Read the model definition and answer for the solid it produces. Units are mm, in the model's axes. Face numbers are marked on the shaded views. A direction names the side the tool comes from. Give positions to 0.01 mm unless a question says otherwise; leave off trailing zeros. Order: outer loops, then holes, each group sorted by start corner. A loop starts at its lowest first (then second) coordinate and runs counter-clockwise, first axis right, second up. Notation, with made-up numbers: (72, 81.25) -> (120, 81.25) arc R17 cw to (120, 95.25) -> close; hole circle Ø11 at (-38, 47.5). An arc over 180 degrees is marked (long way). Answer as CSV lines item,"result". Start each with the question number.
1) Find section C-C (y = 10). Determine the outline of the cut face in (x, z).
2) Straight lines are drawn through the part: L1, parallel to Z at x = 59.5, y = 3; L2, parallel to Y at x = 30, z = -3.7; L3, parallel to X at y = -18, z = -42.5. For each, find the intervals that lie inside material, in ascending order. Write a range as from..to.
3) The mould has two halves that part along X. Classify the marked faces 4, 5 and 6: +X half, -X half, draft (parallel to the pull), parting line (faces both ways), or undercut.
4) Find section D-D (x = 75). State how many separate pieces and enclosed holes the cut face has, and give its area (3 significant figures).
5) Find section B-B (z = -98.5). Determine the outline of the cut face in (x, y), and give its area (3 significant figures).
6) Find section A-A (y = 0). Determine the outline of the cut face in (x, z), and give its area (3 significant figures).
7) For the marked faces 1, 2 and 3, determine the directions among +Z, -Z, +X, -X, +Y, -Y from which every point of the face is accessible in a straight line to the end or side of a thin tool.
8) Flat-ended cylindrical pins translate along their axes: pin 1 Ø2.5 at (x, y) = (3.5, -7) entering from -Z; pin 2 Ø13.5 at (y, z) = (-7, -70.5) entering from +X; pin 3 Ø4 at (y, z) = (8.5, -46) entering from -X. Find the tip coordinate at first contact, or state that the pin passes through.
```python
from build123d import *

# Parameters (mm, degrees)
SKETCH1_W           = 65
SKETCH1_H           = 162
BOSS_EXTRUDE1_DEPTH = 42.5
CUT_EXTRUDE1_DEPTH  = 206.949629764
CUT_EXTRUDE2_REACH  = 207.95
SKETCH4_R           = 4.25
SKETCH5_W           = 2
SKETCH5_H           = 65
CUT_EXTRUDE3_DEPTH  = 206.949629919
CHAMFER1_SIZE       = 20


with BuildPart() as part:
    # Sketch1 → Boss-Extrude1 (new, symmetric)
    with BuildSketch(Plane(origin=(0, 0, 0), x_dir=(1, 0, 0), z_dir=(0, 1, 0))):
        Polygon((100, 5), (100, 167), (105, 172), (0, 172), (5, 167), (5, 5), (0, 5), (0, 0), (105, 0), (105, 5), align=None)
        with Locations((52.5, 86)):
            Rectangle(SKETCH1_W, SKETCH1_H, mode=Mode.SUBTRACT)
    extrude(amount=BOSS_EXTRUDE1_DEPTH, both=True)

    # Sketch2 → Cut-Extrude1 (cut, through all)
    with BuildSketch(Plane(origin=(0, 0, 0), x_dir=(0, 0, -1), z_dir=(1, 0, 0))):
        Polygon((0, 22.5), (147, 22.5), (167, 42.5), (0, 42.5), align=None)
    cut_extrude1 = extrude(amount=CUT_EXTRUDE1_DEPTH, mode=Mode.SUBTRACT)

    # Mirror1: Cut-Extrude1 across plane
    add(cut_extrude1.mirror(Plane.ZX), mode=Mode.SUBTRACT)

    # Sketch3 → section 0 of cut_loft1
    with BuildSketch(Plane(origin=(0, 0, -170), x_dir=(-1, 0, 0), z_dir=(0, 0, -1)), mode=Mode.PRIVATE) as cut_loft1_s0:
        with BuildLine():
            Line((-102.5, 40), (0, 40))
            Line((0, 40), (0, -40))
            Line((0, -40), (-102.5, -40))
            Line((-102.5, -40), (-102.5, 40))
        make_face()
    # loft up to a face of the part (cut_loft1)
    loft([cut_loft1_s0.sketch, part.faces().sort_by_distance((52.5, 0, -172))[0]], mode=Mode.SUBTRACT)

    # Sketch4 → Cut-Extrude2 (cut, up to next)
    with BuildSketch(Plane.XY, mode=Mode.PRIVATE) as cut_extrude2_sk1:
        with Locations((30, 0)):
            Circle(SKETCH4_R)
    cut_extrude2_tool1 = extrude(cut_extrude2_sk1.sketch, amount=-CUT_EXTRUDE2_REACH, mode=Mode.PRIVATE) & part.part
    # Sketch4 → Cut-Extrude2 (cut, up to next)
    with BuildSketch(Plane.XY, mode=Mode.PRIVATE) as cut_extrude2_sk2:
        with Locations((75, 0)):
            Circle(SKETCH4_R)
    cut_extrude2_tool2 = extrude(cut_extrude2_sk2.sketch, amount=-CUT_EXTRUDE2_REACH, mode=Mode.PRIVATE) & part.part
    add(cut_extrude2_tool1.solids().sort_by_distance((30, 0, 0))[0], mode=Mode.SUBTRACT)
    add(cut_extrude2_tool2.solids().sort_by_distance((75, 0, 0))[0], mode=Mode.SUBTRACT)

    # Sketch5 → Cut-Extrude3 (cut, through all)
    with BuildSketch(Plane(origin=(0, 0, 0), x_dir=(0, 0, -1), z_dir=(1, 0, 0))):
        with Locations((171, 0)):
            Rectangle(SKETCH5_W, SKETCH5_H)
    extrude(amount=CUT_EXTRUDE3_DEPTH, mode=Mode.SUBTRACT)

    # Chamfer1
    chamfer1_edges = [part.edges().sort_by_distance(p)[0] for p in [
        (85, 0, -167),
        (20, 0, -167),
    ]]
    chamfer(chamfer1_edges, length=CHAMFER1_SIZE)


solid = part.part
```
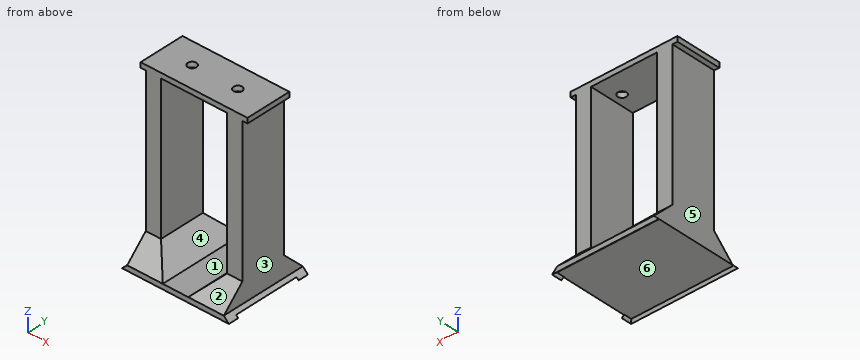
Findings below:
1,outline,"(0, -5) -> (5, -5) -> (5, -167) -> (2, -170) -> (103, -170) -> (100, -167) -> (100, -5) -> (105, -5) -> (105, 0) -> (0, 0) -> close; hole (20, -147) -> (40, -167) -> (65, -167) -> (85, -147) -> (85, -5) -> (20, -5) -> close"
2,L1,"-170..-167, -5..0"
2,L2,"-22.5..-4.25, 4.25..22.5"
2,L3,"5..20, 85..100"
3,face 4,"undercut"
3,face 5,"-X half"
3,face 6,"draft"
4,separate pieces,"3"
4,enclosed holes,"0"
4,area,"1,190 mm²"
5,outline,"(5, -22.5) -> (20, -22.5) -> (20, 22.5) -> (5, 22.5) -> close; (85, -22.5) -> (100, -22.5) -> (100, 22.5) -> (85, 22.5) -> close"
5,area,"1,350 mm²"
6,outline,"(0, -5) -> (5, -5) -> (5, -167) -> (2, -170) -> (103, -170) -> (100, -167) -> (100, -5) -> (105, -5) -> (105, 0) -> (79.25, 0) -> (79.25, -5) -> (85, -5) -> (85, -147) -> (65, -167) -> (40, -167) -> (20, -147) -> (20, -5) -> (25.75, -5) -> (25.75, 0) -> (0, 0) -> close; (34.25, -5) -> (70.75, -5) -> (70.75, 0) -> (34.25, 0) -> close"
6,area,"5,990 mm²"
7,face 1,"+Y, -Y"
7,face 2,"+Z, +X, -X, -Y"
7,face 3,"+X, +Y, -Y"
8,pin 1,"z = -170"
8,pin 2,"x = 100"
8,pin 3,"x = 5"
